from build123d import *

# Parameters (mm, degrees)
SKETCH1_W           = 98
SKETCH1_H           = 25
BOSS_EXTRUDE1_DEPTH = 10
CUT_EXTRUDE4_DEPTH  = 10
SKETCH4_W           = 25
SKETCH4_H           = 10
CUT_EXTRUDE6_DEPTH  = 5
SKETCH5_W           = 25
SKETCH5_H           = 10
CUT_EXTRUDE7_DEPTH  = 5
SKETCH6_W           = 5
SKETCH6_H           = 10
CUT_EXTRUDE8_DEPTH  = 5
SKETCH7_W           = 5
SKETCH7_H           = 10
CUT_EXTRUDE9_DEPTH  = 5
CUT_EXTRUDE10_DEPTH = 1.5
SKETCH9_R           = 1
CUT_EXTRUDE11_DEPTH = 11.5
SKETCH10_R          = 1
CUT_EXTRUDE12_DEPTH = 19.5
SKETCH11_R          = 1.75
CUT_EXTRUDE13_DEPTH = 1.5


with BuildPart() as part:
    # Sketch1 → Boss-Extrude1 (new body)
    with BuildSketch(Plane(origin=(0, 0, 0), x_dir=(1, 0, 0), z_dir=(0, 1, 0))):
        Rectangle(SKETCH1_W, SKETCH1_H)
    extrude(amount=BOSS_EXTRUDE1_DEPTH)

    # Sketch2 → Cut-Extrude4 (cut)
    with BuildSketch(Plane(origin=(0, 10, 0), x_dir=(1, 0, 0), z_dir=(0, 1, 0))):
        Polygon((-2.5, 2.403992328), (-2.5, -7.5), (-34, -7.5), (-34, 7.5), (-2.5, 7.5), align=None)
        Polygon((2.5, 2.403992328), (2.5, 7.5), (34, 7.5), (34, -7.5), (2.5, -7.5), align=None)
    extrude(amount=-CUT_EXTRUDE4_DEPTH, mode=Mode.SUBTRACT)

    # Sketch4 → Cut-Extrude6 (cut)
    with BuildSketch(Plane.ZY.offset(49)):
        with Locations((0, 5)):
            Rectangle(SKETCH4_W, SKETCH4_H)
    extrude(amount=-CUT_EXTRUDE6_DEPTH, mode=Mode.SUBTRACT)

    # Sketch5 → Cut-Extrude7 (cut)
    with BuildSketch(Plane(origin=(49, 0, 0), x_dir=(0, 0, -1), z_dir=(1, 0, 0))):
        with Locations((0, 5)):
            Rectangle(SKETCH5_W, SKETCH5_H)
    extrude(amount=-CUT_EXTRUDE7_DEPTH, mode=Mode.SUBTRACT)

    # Sketch6 → Cut-Extrude8 (cut)
    with BuildSketch(Plane(origin=(44, 0, 0), x_dir=(0, 0, -1), z_dir=(1, 0, 0))):
        with Locations((0, 5)):
            Rectangle(SKETCH6_W, SKETCH6_H)
    extrude(amount=-CUT_EXTRUDE8_DEPTH, mode=Mode.SUBTRACT)

    # Sketch7 → Cut-Extrude9 (cut)
    with BuildSketch(Plane.ZY.offset(44)):
        with Locations((0, 5)):
            Rectangle(SKETCH7_W, SKETCH7_H)
    extrude(amount=-CUT_EXTRUDE9_DEPTH, mode=Mode.SUBTRACT)

    # Sketch8 → Cut-Extrude10 (cut)
    with BuildSketch(Plane.XZ):
        with BuildLine():
            ThreePointArc((0, 11.75), (-1.75, 10), (0, 8.25))
            Line((0, 8.25), (0, 11.75))
        make_face()
        with BuildLine():
            Line((0, 11.75), (0, 8.25))
            ThreePointArc((0, 8.25), (1.237436867, 8.762563133), (1.75, 10))
            ThreePointArc((1.75, 10), (1.237436867, 11.237436867), (0, 11.75))
        make_face()
    extrude(amount=-CUT_EXTRUDE10_DEPTH, mode=Mode.SUBTRACT)

    # Sketch9 → Cut-Extrude11 (cut)
    with BuildSketch(Plane.XZ.offset(-1.5)):
        with Locations(Location((0, 10, 0), (0, 0, 270))):
            Circle(SKETCH9_R)
    extrude(amount=-CUT_EXTRUDE11_DEPTH, mode=Mode.SUBTRACT)

    # Sketch10 → Cut-Extrude12 (cut)
    with BuildSketch(Plane.XZ):
        with Locations(Location((0, -10.129347353, 0), (0, 0, 270))):
            Circle(SKETCH10_R)
    extrude(amount=-CUT_EXTRUDE12_DEPTH, mode=Mode.SUBTRACT)

    # Sketch11 → Cut-Extrude13 (cut)
    with BuildSketch(Plane.XZ):
        with Locations(Location((0, -10.129347353, 0), (0, 0, 270))):
            Circle(SKETCH11_R)
    extrude(amount=-CUT_EXTRUDE13_DEPTH, mode=Mode.SUBTRACT)


solid = part.part
Source: CAD feature listing. Evaluate the final solid. Frame: model axes, mm. A direction names the side the tool comes from. Round coordinates to 2 decimals unless told otherwise and drop trailing zeros. Order: outer loops, then holes, each group sorted by start corner. A loop starts at its lowest first (then second) coordinate and runs counter-clockwise, first axis right, second up. Notation, with made-up numbers: (-35, -7.5) - (3, -7.5) arc R21 cw to (3, 5.5) - close; hole circle Ø10 at (31.5, 75). An arc over 180 degrees is marked (long way). Use a Markdown table: item, result. Add a question column.
1. Mould query, pull axis Z, two halves, no side actions, for faces 1 (the flat face through (-1, 5, -12.5)), 2 (the flat face through (44, 5, -7)), 3 (the cylindrical face through (-0.6, 5.7, 10.8)). Classes: +Z half, -Z half, draft (parallel to the pull), parting line (faces both ways), or undercut.
2. Section query A-A (z = 0.5). Return the cut outline in (x, y).
3. Set-up query: faces 4 (the flat face through (-2.5, 5, 0)), 5 (the flat face through (-1, 1.5, -11)), 6 (the flat face through (-39, 5, 0)). Return all of +Z, -Z, +X, -X, +Y, -Y with unobstructed straight access to the full face (end or side cutting, diameter ignored); none if empty.
4. First-contact query: pin 1 (2.5 mm diameter, centred on y = 6, z = -1, fed in from -X); pin 2 (1.6 mm diameter, centred on x = 0, z = 10, fed in from -Y); pin 3 (1.8 mm diameter, centred on x = -0.5, z = -10, fed in from -Y). Flat tips, straight axial feed; report the tip coordinate or a pass-through.
5. Section query D-D (z = 6.5). Return the cut outline in (x, y).
6. Section query C-C (y = 4.5). Return the cut outline in (x, z).
7. Line query: probe 1 along X at (y, z) = (5.5, 4.5); probe 2 along X at (y, z) = (1.5, -1.75); probe 3 along X at (y, z) = (5.25, 10). Output: solid intervals per line, ascending.
8. Section query B-B (x = 30). Return the cut outline in (y, z), then the cut area to 3 significant figures.
Derived:
| question | item | result |
|---|---|---|
| 1 | face 1 | -Z half |
| 1 | face 2 | draft |
| 1 | face 3 | undercut |
| 2 | outline | (-39, 0) - (-34, 0) - (-34, 10) - (-39, 10) - close; (-2.5, 0) - (2.5, 0) - (2.5, 10) - (-2.5, 10) - close; (34, 0) - (39, 0) - (39, 10) - (34, 10) - close |
| 3 | face 4 | +Y, -Y |
| 3 | face 5 | -Y |
| 3 | face 6 | -X, +Y, -Y |
| 4 | pin 1 | x = -39 |
| 4 | pin 2 | through |
| 4 | pin 3 | y = 1.5 |
| 5 | outline | (-44, 0) - (-34, 0) - (-34, 10) - (-44, 10) - close; (-2.5, 0) - (2.5, 0) - (2.5, 10) - (-2.5, 10) - close; (34, 0) - (44, 0) - (44, 10) - (34, 10) - close |
| 6 | outline | (-44, -12.5) - (44, -12.5) - (44, -2.5) - (39, -2.5) - (39, 2.5) - (44, 2.5) - (44, 12.5) - (-44, 12.5) - (-44, 2.5) - (-39, 2.5) - (-39, -2.5) - (-44, -2.5) - close; hole (-34, -7.5) - (-2.5, -7.5) - (-2.5, 7.5) - (-34, 7.5) - close; hole circle Ø2 at (0, -10.13); hole circle Ø2 at (0, 10); hole (2.5, -7.5) - (34, -7.5) - (34, 7.5) - (2.5, 7.5) - close |
| 7 | probe 1 | -44 to -34, -2.5 to 2.5, 34 to 44 |
| 7 | probe 2 | -39 to -34, -2.5 to 2.5, 34 to 39 |
| 7 | probe 3 | -44 to -1, 1 to 44 |
| 8 | outline | (0, -12.5) - (10, -12.5) - (10, -7.5) - (0, -7.5) - close; (0, 7.5) - (10, 7.5) - (10, 12.5) - (0, 12.5) - close |
| 8 | area | 100 mm2 |
